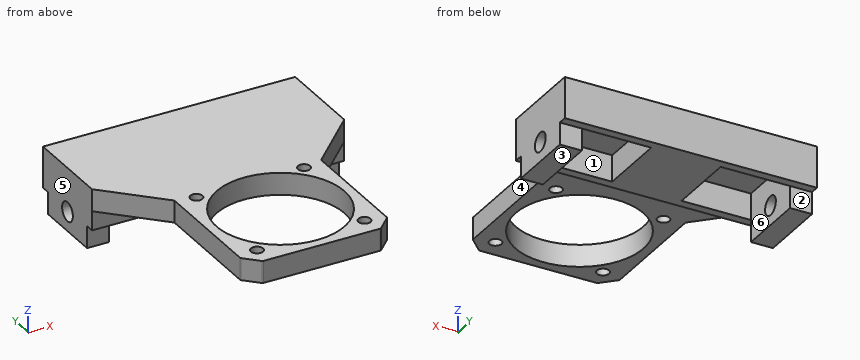
Autodesk Inventor part; units mm, degrees
ref_plane "YZ Plane" through (0, 0, 0) normal (1, 0, 0) x (0, 1, 0)
ref_plane "XZ Plane" through (0, 0, 0) normal (0, 1, 0) x (-1, 0, 0)
ref_plane "XY Plane" through (0, 0, 0) normal (0, 0, 1) x (1, 0, 0)
sketch "Sketch1" plane through (0, 0, 0) normal (0, 0, 1) x (1, 0, 0)
  circle A0 centre (-40, 0) radius 2.5
  arc A1 (-31.25, -10) -> (-30, -8.75) centre (-31.25, -8.75) ccw
  line L0 (-30, -3.6) -> (-30, -8.75)
  line L1 (-30.5, -3.1) -> (-30, -3.6)
  line L2 (-31.6, -3.1) -> (-30.5, -3.1)
  line L3 (-31.6, -5.5) -> (-31.6, -3.1)
  line L4 (-33.534, -5.5) -> (-31.6, -5.5)
  line L5 (-35.9, -3.134) -> (-33.534, -5.5)
  line L6 (-35.9, 3.134) -> (-35.9, -3.134)
  line L7 (-33.534, 5.5) -> (-35.9, 3.134)
  line L8 (-31.6, 5.5) -> (-33.534, 5.5)
  line L9 (-31.6, 3.1) -> (-31.6, 5.5)
  line L10 (-30.5, 3.1) -> (-31.6, 3.1)
  line L11 (-30, 3.6) -> (-30.5, 3.1)
  line L12 (-30, 8.75) -> (-30, 3.6)
  arc A2 (-30, 8.75) -> (-31.25, 10) centre (-31.25, 8.75) ccw
  line L13 (-36.4, 10) -> (-31.25, 10)
  line L14 (-36.9, 9.5) -> (-36.4, 10)
  line L15 (-36.9, 8.4) -> (-36.9, 9.5)
  line L16 (-34.5, 8.4) -> (-36.9, 8.4)
  line L17 (-34.5, 6.466) -> (-34.5, 8.4)
  line L18 (-36.866, 4.1) -> (-34.5, 6.466)
  line L19 (-43.134, 4.1) -> (-36.866, 4.1)
  line L20 (-45.5, 6.466) -> (-43.134, 4.1)
  line L21 (-45.5, 8.4) -> (-45.5, 6.466)
  line L22 (-43.1, 8.4) -> (-45.5, 8.4)
  line L23 (-43.1, 9.5) -> (-43.1, 8.4)
  line L24 (-43.6, 10) -> (-43.1, 9.5)
  line L25 (-48.75, 10) -> (-43.6, 10)
  arc A3 (-48.75, 10) -> (-50, 8.75) centre (-48.75, 8.75) ccw
  line L26 (-50, 3.6) -> (-50, 8.75)
  line L27 (-49.5, 3.1) -> (-50, 3.6)
  line L28 (-48.4, 3.1) -> (-49.5, 3.1)
  line L29 (-48.4, 5.5) -> (-48.4, 3.1)
  line L30 (-46.466, 5.5) -> (-48.4, 5.5)
  line L31 (-44.1, 3.134) -> (-46.466, 5.5)
  line L32 (-44.1, -3.134) -> (-44.1, 3.134)
  line L33 (-46.466, -5.5) -> (-44.1, -3.134)
  line L34 (-48.4, -5.5) -> (-46.466, -5.5)
  line L35 (-48.4, -3.1) -> (-48.4, -5.5)
  line L36 (-49.5, -3.1) -> (-48.4, -3.1)
  line L37 (-50, -3.6) -> (-49.5, -3.1)
  line L38 (-50, -8.75) -> (-50, -3.6)
  arc A4 (-50, -8.75) -> (-48.75, -10) centre (-48.75, -8.75) ccw
  line L39 (-43.6, -10) -> (-48.75, -10)
  line L40 (-43.1, -9.5) -> (-43.6, -10)
  line L41 (-43.1, -8.4) -> (-43.1, -9.5)
  line L42 (-45.5, -8.4) -> (-43.1, -8.4)
  line L43 (-45.5, -6.466) -> (-45.5, -8.4)
  line L44 (-43.134, -4.1) -> (-45.5, -6.466)
  line L45 (-36.866, -4.1) -> (-43.134, -4.1)
  line L46 (-34.5, -6.466) -> (-36.866, -4.1)
  line L47 (-34.5, -8.4) -> (-34.5, -6.466)
  line L48 (-36.9, -8.4) -> (-34.5, -8.4)
  line L49 (-36.9, -9.5) -> (-36.9, -8.4)
  line L50 (-36.4, -10) -> (-36.9, -9.5)
  line L51 (-31.25, -10) -> (-36.4, -10)
  circle A5 centre (0, 0) radius 2.5
  arc A6 (8.75, -10) -> (10, -8.75) centre (8.75, -8.75) ccw
  line L52 (10, -3.6) -> (10, -8.75)
  line L53 (9.5, -3.1) -> (10, -3.6)
  line L54 (8.4, -3.1) -> (9.5, -3.1)
  line L55 (8.4, -5.5) -> (8.4, -3.1)
  line L56 (6.466, -5.5) -> (8.4, -5.5)
  line L57 (4.1, -3.134) -> (6.466, -5.5)
  line L58 (4.1, 3.134) -> (4.1, -3.134)
  line L59 (6.466, 5.5) -> (4.1, 3.134)
  line L60 (8.4, 5.5) -> (6.466, 5.5)
  line L61 (8.4, 3.1) -> (8.4, 5.5)
  line L62 (9.5, 3.1) -> (8.4, 3.1)
  line L63 (10, 3.6) -> (9.5, 3.1)
  line L64 (10, 8.75) -> (10, 3.6)
  arc A7 (10, 8.75) -> (8.75, 10) centre (8.75, 8.75) ccw
  line L65 (3.6, 10) -> (8.75, 10)
  line L66 (3.1, 9.5) -> (3.6, 10)
  line L67 (3.1, 8.4) -> (3.1, 9.5)
  line L68 (5.5, 8.4) -> (3.1, 8.4)
  line L69 (5.5, 6.466) -> (5.5, 8.4)
  line L70 (3.134, 4.1) -> (5.5, 6.466)
  line L71 (-3.134, 4.1) -> (3.134, 4.1)
  line L72 (-5.5, 6.466) -> (-3.134, 4.1)
  line L73 (-5.5, 8.4) -> (-5.5, 6.466)
  line L74 (-3.1, 8.4) -> (-5.5, 8.4)
  line L75 (-3.1, 9.5) -> (-3.1, 8.4)
  line L76 (-3.6, 10) -> (-3.1, 9.5)
  line L77 (-8.75, 10) -> (-3.6, 10)
  arc A8 (-8.75, 10) -> (-10, 8.75) centre (-8.75, 8.75) ccw
  line L78 (-10, 3.6) -> (-10, 8.75)
  line L79 (-9.5, 3.1) -> (-10, 3.6)
  line L80 (-8.4, 3.1) -> (-9.5, 3.1)
  line L81 (-8.4, 5.5) -> (-8.4, 3.1)
  line L82 (-6.466, 5.5) -> (-8.4, 5.5)
  line L83 (-4.1, 3.134) -> (-6.466, 5.5)
  line L84 (-4.1, -3.134) -> (-4.1, 3.134)
  line L85 (-6.466, -5.5) -> (-4.1, -3.134)
  line L86 (-8.4, -5.5) -> (-6.466, -5.5)
  line L87 (-8.4, -3.1) -> (-8.4, -5.5)
  line L88 (-9.5, -3.1) -> (-8.4, -3.1)
  line L89 (-10, -3.6) -> (-9.5, -3.1)
  line L90 (-10, -8.75) -> (-10, -3.6)
  arc A9 (-10, -8.75) -> (-8.75, -10) centre (-8.75, -8.75) ccw
  line L91 (-3.6, -10) -> (-8.75, -10)
  line L92 (-3.1, -9.5) -> (-3.6, -10)
  line L93 (-3.1, -8.4) -> (-3.1, -9.5)
  line L94 (-5.5, -8.4) -> (-3.1, -8.4)
  line L95 (-5.5, -6.466) -> (-5.5, -8.4)
  line L96 (-3.134, -4.1) -> (-5.5, -6.466)
  line L97 (3.134, -4.1) -> (-3.134, -4.1)
  line L98 (5.5, -6.466) -> (3.134, -4.1)
  line L99 (5.5, -8.4) -> (5.5, -6.466)
  line L100 (3.1, -8.4) -> (5.5, -8.4)
  line L101 (3.1, -9.5) -> (3.1, -8.4)
  line L102 (3.6, -10) -> (3.1, -9.5)
  line L103 (8.75, -10) -> (3.6, -10)
  line L104 (-50, -10) -> (-50, 10)
  line L105 (10, 10) -> (10, -10)
  line L106 (-30, -10) -> (-30, 10)
  line L107 (-10, 10) -> (-10, -10)
  line L108 (-52.54, -12.54) -> (12.54, -12.54)
  line L109 (12.54, -12.54) -> (12.54, 12.54)
  line L110 (12.54, 12.54) -> (-52.54, 12.54)
  line L111 (-52.54, 12.54) -> (-52.54, -12.54)
  line L112 (10, -10) -> (-10, -10)
  line L113 (-30, -10) -> (-50, -10)
  line L114 (-50, 10) -> (-30, 10)
  line L115 (-10, 10) -> (10, 10)
  point P0 (0, 0)
extrude "Extrusion1" add sketch "Sketch1" against normal blind 7.62 contours L111 L110 L109 L108
sketch "Sketch2" plane through (0, 0, 0) normal (0, 0, 1) x (1, 0, 0)
  line L0 (-52.54, -12.54) -> (-52.54, 12.54)
  line L1 (12.54, -12.54) -> (12.54, 12.54)
  line L2 (-52.54, -12.54) -> (12.54, -12.54)
  line L3 (12.54, -12.54) -> (12.54, 12.54)
  line L4 (12.54, 12.54) -> (-52.54, 12.54)
  line L5 (-52.54, 12.54) -> (-52.54, -12.54)
  point P0 (0, 0)
extrude "Extrusion2" add sketch "Sketch2" along normal blind 4.25
sketch "Sketch4" plane through (0, 0, 4.25) normal (0, 0, 1) x (1, 0, 0)
  line L0 (-52.54, -12.54) -> (12.54, -12.54)
  line L1 (12.54, -12.54) -> (12.54, 12.54)
  line L2 (12.54, 12.54) -> (-52.54, 12.54)
  line L3 (-52.54, 12.54) -> (-52.54, -12.54)
  line L4 (-36.8267, -23.35) -> (-3.1733, -23.35)
  arc A0 (-2.8198, -23.4964) -> (-3.1733, -23.35) centre (-3.1733, -23.85) ccw
  line L5 (-2.8198, -23.4964) -> (1.0036, -27.3198)
  arc A1 (1.15, -27.6733) -> (1.0036, -27.3198) centre (0.65, -27.6733) ccw
  line L6 (1.15, -27.6733) -> (1.15, -61.3267)
  arc A2 (1.0036, -61.6802) -> (1.15, -61.3267) centre (0.65, -61.3267) ccw
  line L7 (1.0036, -61.6802) -> (-2.8198, -65.5036)
  arc A3 (-3.1733, -65.65) -> (-2.8198, -65.5036) centre (-3.1733, -65.15) ccw
  line L8 (-3.1733, -65.65) -> (-36.8267, -65.65)
  arc A4 (-37.1802, -65.5036) -> (-36.8267, -65.65) centre (-36.8267, -65.15) ccw
  line L9 (-37.1802, -65.5036) -> (-41.0036, -61.6802)
  arc A5 (-41.15, -61.3267) -> (-41.0036, -61.6802) centre (-40.65, -61.3267) ccw
  line L10 (-41.15, -61.3267) -> (-41.15, -27.6733)
  arc A6 (-41.0036, -27.3198) -> (-41.15, -27.6733) centre (-40.65, -27.6733) ccw
  line L11 (-41.0036, -27.3198) -> (-37.1802, -23.4964)
  arc A7 (-36.8267, -23.35) -> (-37.1802, -23.4964) centre (-36.8267, -23.85) ccw
  circle A8 centre (-4.5, -29) radius 1.75
  circle A9 centre (-35.5, -29) radius 1.75
  circle A10 centre (-35.5, -60) radius 1.75
  circle A11 centre (-4.5, -60) radius 1.75
  circle A12 centre (-20, -44.5) radius 17
  line L12 (-41.15, -27.6733) -> (-41.15, -12.54)
  line L13 (-51.3494, -12.54) -> (11.3494, -12.54)
  line L14 (1.15, -27.6733) -> (1.15, -12.54)
  circle A13 centre (-20, -44.5) radius 18.4562
  point P0 (0, 0)
extrude "Extrusion3" add sketch "Sketch4" against normal blind 6.35 contours L0 L14 A1 L5 A0 L4 A7 L11 A6 L12 | A6 L11 A7 L4 A0 L5 A1 L6 A2 L7 A3 L8 A4 L9 A5 L10
sketch "Sketch7" plane through (12.54, -12.54, -7.62) normal (1, 0, 0) x (0, 0, -1)
  line L0 (-7.62, 22.54) -> (-7.62, 2.54)
  line L1 (0, 0) -> (-11.87, 0)
  line L2 (0, 25.08) -> (0, 0)
  line L3 (0, 25.08) -> (-11.87, 25.08)
  line L4 (-11.87, 0) -> (-11.87, 25.08)
  point P0 (-7.62, 12.54)
extrude "Extrusion5" add sketch "Sketch7" along normal blind 3.81
sketch "Sketch8" plane through (-52.54, -12.54, -7.62) normal (-1, 0, 0) x (0, 0, 1)
  line L0 (0, 25.08) -> (11.87, 25.08)
  line L1 (0, 0) -> (0, 25.08)
  line L2 (11.87, 0) -> (0, 0)
  line L3 (11.87, 25.08) -> (11.87, 0)
  point P0 (7.62, 12.54)
extrude "Extrusion6" add sketch "Sketch8" along normal blind 3.81
sketch "Sketch9" plane through (0, 0, -2.1) normal (0, 0, -1) x (-1, 0, 0)
  line L0 (-1.15, -12.54) -> (-16.35, -12.54)
  line L1 (-16.35, -12.54) -> (-1.15, -27.74)
  line L2 (56.35, -12.54) -> (56.35, 12.54)
  line L3 (56.35, -12.54) -> (41.15, -27.74)
  line L4 (41.15, -12.54) -> (41.15, -61.3267)
  line L5 (-1.15, -12.54) -> (-1.15, -61.3267)
  line L6 (-1.15, -12.54) -> (41.15, -12.54)
  line L7 (41.15, -12.54) -> (56.35, -12.54)
  line L8 (41.15, -12.54) -> (56.35, -12.54)
  line L9 (41.15, -12.54) -> (41.15, -27.74)
  line L10 (-1.15, -61.3267) -> (-1.15, -12.54)
  line L11 (-1.15, -27.74) -> (-1.15, -12.54)
  line L12 (-1.15, -12.54) -> (-16.35, -12.54)
  point P0 (0, 0)
  dimension "d16" = 45
  dimension "d17" = 45
extrude "Extrusion7" add sketch "Sketch9" against normal up to surface (6.35 mm away)
sketch "Sketch10" plane through (0, 0, -7.62) normal (0, 0, -1) x (-1, 0, 0)
  line L0 (-16.35, 12.54) -> (-16.35, -12.54)
  line L1 (-10, 10) -> (-10, -10)
  line L2 (-10, -10) -> (-16.35, -10)
  line L3 (-16.35, -10) -> (-16.35, 10)
  line L4 (56.35, 12.54) -> (56.35, -12.54)
  line L5 (50, 10) -> (50, -10)
  line L6 (50, -10) -> (56.35, -10)
  line L7 (56.35, -10) -> (56.35, 10)
  line L8 (-10, -10) -> (-10, 10)
  line L9 (50, 10) -> (50, -10)
  line L10 (10, -10) -> (-10, -10)
  line L11 (-10, 10) -> (10, 10)
  line L12 (-10, 10) -> (-16.35, 10)
  line L13 (30, 10) -> (50, 10)
  line L14 (50, 10) -> (56.35, 10)
  point P0 (0, 0)
  dimension "d20" = 0
  dimension "d21" = 0
  dimension "d30" = 0
extrude "Extrusion8" add sketch "Sketch10" along normal blind 6.35
sketch "Sketch11" plane through (-56.35, -12.54, -7.62) normal (-1, 0, 0) x (0, 0, 1)
  line L0 (5.52, 2.54) -> (-6.35, 2.54)
  line L1 (-6.35, 2.54) -> (15.282, 2.54)
  line L2 (-6.35, 2.54) -> (-6.35, 22.54)
  line L3 (-6.35, 22.54) -> (2.1036, 22.54)
  line L4 (7.62, 22.54) -> (0, 22.54)
  circle A0 centre (-0.7499, 12.54) radius 2.75
  line L5 (-0.7499, 12.54) -> (-0.7499, 22.54)
  line L6 (-0.7499, 12.54) -> (-0.7499, 2.54)
  line L7 (0, 2.54) -> (-6.35, 2.54)
  point P0 (7.62, 12.54)
  point P1 (5.52, 0)
  dimension "d32" = 5.5
extrude "Extrusion9" cut sketch "Sketch11" against normal through all contours L6 L5 A0 | A0 L5 L6
sketch "Sketch12" plane through (-30, -10, 0) normal (-1, 0, 0) x (0, 0, 1)
  arc A0 (-7.62, 7.3542) -> (-7.62, 12.6458) centre (-8.3699, 10) ccw
  line L0 (-7.62, 7.3542) -> (-7.62, 12.6458)
  point P0 (0, 10)
extrude "Extrusion10" add sketch "Sketch12" against normal up to surface (20 mm away)
properties part number "motorBracketY"
CAD build for the part. Positions are in the model's coordinates, mm. Face numbers are marked on the shaded views. A direction names the side the tool comes from. Round coordinates to 2 decimals unless told otherwise and drop trailing zeros. Loops run counter-clockwise (first coordinate to the right, second up) from the corner with the lowest first, then second, coordinate; pieces in that order, holes last. Notation, with made-up numbers: (88.25, 15) - (146.25, 15) arc R25 cw to (146.25, 35) - close; hole circle Ø8 at (24, 59). An arc over 180 degrees is marked (long way). Return JSON: item names as keys, results as strings. Group by question number.
Q1. Band-saw the part on D-D on x = -35. Give the cut face in (y, z), plus the area to 3 significant figures.
Q2. Band-saw the part on A-A on y = 0. Give the cut face in (x, z).
Q3. Drill centre lines: line 1 along X through (y, z) = (2.5, -12.75); line 2 along Y through (x, z) = (-4.5, 2.25); line 3 along Z through (x, y) = (-24, -4). Where is each one in solid material? Low to high. Write a range as [from, to].
Q4. Band-saw the part on C-C on y = -44.5. Give the cut face in (x, z), plus the area to 3 significant figures.
Q5. Flat gauge pins, fed straight in: pin 1 Ø3 at (x, z) = (-53, -12) entering from -Y; pin 2 Ø2 at (x, y) = (-35.5, -60) entering from -Z; pin 3 Ø1 at (x, z) = (-2.5, -3) entering from -Y; pin 4 Ø6 at (x, y) = (-5, -2.5) entering from -Z. Where does each tip first touch, or does it go through?
Q6. Tool access for the marked faces 1, 2 and 3: list every direction of +Z, -Z, +X, -X, +Y, -Y with a clear straight run to the whole face (end or side of a thin tool).
Q7. Two-plate mould, pull along X, no slides. Class the marked faces 4, 5 and 6: +X half, -X half, draft (parallel to the pull), parting line (faces both ways), or undercut.
Q8. Band-saw the part on B-B on z = 3. Give the cut face in (x, y), plus the area to 3 significant figures.
Solutions:
{
 "1": {"outline": "(-65.65, -2.1) - (-61.68, -2.1) - (-61.68, 4.25) - (-65.65, 4.25) - close; (-58.32, -2.1) - (-55.25, -2.1) - (-55.25, 4.25) - (-58.32, 4.25) - close; (-33.75, -2.1) - (-30.68, -2.1) - (-30.68, 4.25) - (-33.75, 4.25) - close; (-27.32, -2.1) - (-12.54, -2.1) - (-12.54, -7.62) - (-10, -7.62) - (-10, 0) - (10, 0) - (10, -7.62) - (12.54, -7.62) - (12.54, 4.25) - (-27.32, 4.25) - close", "area": "303 mm^2"},
 "2": {"outline": "(-56.35, -13.97) - (-50, -13.97) - (-50, -11.12) - (-56.35, -11.12) - close; (-56.35, -5.62) - (-50, -5.62) - (-50, 0) - (-30, 0) - (-30, -7.62) - (-10, -7.62) - (-10, 0) - (10, 0) - (10, -5.62) - (16.35, -5.62) - (16.35, 4.25) - (-56.35, 4.25) - close; (10, -13.97) - (16.35, -13.97) - (16.35, -11.12) - (10, -11.12) - close"},
 "3": {"line 1": "x = [-56.35, -50], [10, 16.35]", "line 2": "y = [-65.65, -61.75], [-58.25, -54.52], [-34.48, -30.75], [-27.25, 12.54]", "line 3": "z = [-7.62, 4.25]"},
 "4": {"outline": "(-41.15, -2.1) - (-38.46, -2.1) - (-38.46, 4.25) - (-41.15, 4.25) - close; (-1.54, -2.1) - (1.15, -2.1) - (1.15, 4.25) - (-1.54, 4.25) - close", "area": "34.2 mm^2"},
 "5": {"pin 1": "stops at y = -10", "pin 2": "passes through", "pin 3": "stops at y = -12.54", "pin 4": "stops at z = 0"},
 "6": {"face 1": "-Z", "face 2": "-Z, +X, -X, +Y", "face 3": "-Z, +X, -X, +Y, -Y"},
 "7": {"face 4": "+X half", "face 5": "-X half", "face 6": "undercut"},
 "8": {"outline": "(-56.35, -12.54) - (-41.15, -27.74) - (-41.15, -61.33) arc R0.5 ccw to (-41, -61.68) - (-37.18, -65.5) arc R0.5 ccw to (-36.83, -65.65) - (-3.17, -65.65) arc R0.5 ccw to (-2.82, -65.5) - (1, -61.68) arc R0.5 ccw to (1.15, -61.33) - (1.15, -27.74) - (16.35, -12.54) - (16.35, 12.54) - (-56.35, 12.54) - close; hole circle Ø36.91 at (-20, -44.5); hole circle Ø3.5 at (-35.5, -60); hole circle Ø3.5 at (-35.5, -29); hole circle Ø3.5 at (-4.5, -60); hole circle Ø3.5 at (-4.5, -29)", "area": "3,180 mm^2"}
}
